Verification items for the finished model (mm, model axes). Give positions to 0.01 mm unless a question says otherwise; leave off trailing zeros. Write each loop counter-clockwise with the first axis right and the second up, starting at its lowest first coordinate (ties: lowest second). Pieces come first, ordered by that corner, then holes.
from build123d import *

# Parameters (mm, degrees)
SKETCH_1_R          = 13
EXTRUDE_1_DEPTH     = 8
SKETCH_6_R          = 14
EXTRUDE_4_DEPTH     = 8
SKETCH_2_R          = 12
CUT_EXTRUDE_1_DEPTH = 3
CUT_EXTRUDE_2_DEPTH = 22.354156504
SKETCH_8_R          = 2.5
CUT_EXTRUDE_3_DEPTH = 2


with BuildPart() as part:
    # 草图1 → 凸台-拉伸1 (new body)
    with BuildSketch(Plane(origin=(0, 0, 0), x_dir=(1, 0, 0), z_dir=(0, 1, 0))):
        with Locations(Location((0, 0, 0), (0, 0, 270))):
            Circle(SKETCH_1_R)
    extrude(amount=EXTRUDE_1_DEPTH)

    # 草图6 → 凸台-拉伸4 (add, through all)
    with BuildSketch(Plane(origin=(0, 8, 0), x_dir=(1, 0, 0), z_dir=(0, 1, 0))):
        with Locations(Location((0, 0, 0), (0, 0, 270))):
            Circle(SKETCH_6_R)
    extrude(amount=-EXTRUDE_4_DEPTH)

    # 草图2 → 切除-拉伸1 (cut)
    with BuildSketch(Plane(origin=(0, 8, 0), x_dir=(1, 0, 0), z_dir=(0, 1, 0))):
        with Locations(Location((0, 0, 0), (0, 0, 270))):
            Circle(SKETCH_2_R)
    extrude(amount=-CUT_EXTRUDE_1_DEPTH, mode=Mode.SUBTRACT)

    # 草图7 → 切除-拉伸2 (cut, through all)
    with BuildSketch(Plane(origin=(0, 8, 0), x_dir=(1, 0, 0), z_dir=(0, 1, 0))):
        Polygon((-15.646830527, 4.142221687), (-12.567085782, 3.326913727), (-12.296421758, 4.349320163), (-15.376166503, 5.164628122), align=None)
        Polygon((-14.689830765, 6.79633564), (-11.798451005, 5.458621977), (-11.354359961, 6.418495447), (-14.245739722, 7.756209109), align=None)
        Polygon((-13.28648793, 9.243946373), (-10.671326264, 7.42447276), (-10.067301683, 8.292647994), (-12.682463348, 10.112121607), align=None)
        Polygon((-11.479441881, 11.410684473), (-9.219958675, 9.164734695), (-8.474353537, 9.914832629), (-10.733836743, 12.160782407), align=None)
        Polygon((-9.3235988, 13.230714699), (-7.488447307, 10.626530804), (-6.623916447, 11.235760092), (-8.45906794, 13.839943987), align=None)
        Polygon((-6.884462888, 14.648736355), (-5.529403257, 11.765445152), (-4.572215008, 12.215294669), (-5.927274639, 15.098585872), align=None)
        Polygon((-4.236146054, 15.621663569), (-3.402351087, 12.546872402), (-2.381589129, 12.8236737), (-3.215384096, 15.898464866), align=None)
        Polygon((-1.459116066, 16.11993444), (-1.171920201, 12.947069284), (-0.11859987, 13.042411894), (-0.405795735, 16.21527705), align=None)
        Polygon((1.362248425, 16.12840926), (1.094118888, 12.953876017), (2.147992986, 12.864863002), (2.416122524, 16.039396246), align=None)
        Polygon((4.142221687, 15.646830527), (3.326913727, 12.567085782), (4.349320163, 12.296421758), (5.164628122, 15.376166503), align=None)
        Polygon((6.79633564, 14.689830765), (5.458621977, 11.798451005), (6.418495447, 11.354359961), (7.756209109, 14.245739722), align=None)
        Polygon((9.243946373, 13.28648793), (7.42447276, 10.671326264), (8.292647994, 10.067301683), (10.112121607, 12.682463348), align=None)
        Polygon((11.410684473, 11.479441881), (9.164734695, 9.219958675), (9.914832629, 8.474353537), (12.160782407, 10.733836743), align=None)
        Polygon((13.230714699, 9.3235988), (10.626530804, 7.488447307), (11.235760092, 6.623916447), (13.839943987, 8.45906794), align=None)
        Polygon((14.648736355, 6.884462888), (11.765445152, 5.529403257), (12.215294669, 4.572215008), (15.098585872, 5.927274639), align=None)
        Polygon((15.621663569, 4.236146054), (12.546872402, 3.402351087), (12.8236737, 2.381589129), (15.898464866, 3.215384096), align=None)
        Polygon((16.11993444, 1.459116066), (12.947069284, 1.171920201), (13.042411894, 0.11859987), (16.21527705, 0.405795735), align=None)
        Polygon((16.12840926, -1.362248425), (12.953876017, -1.094118888), (12.864863002, -2.147992986), (16.039396246, -2.416122524), align=None)
        Polygon((15.646830527, -4.142221687), (12.567085782, -3.326913727), (12.296421758, -4.349320163), (15.376166503, -5.164628122), align=None)
        Polygon((14.689830765, -6.79633564), (11.798451005, -5.458621977), (11.354359961, -6.418495447), (14.245739722, -7.756209109), align=None)
        Polygon((13.28648793, -9.243946373), (10.671326264, -7.42447276), (10.067301683, -8.292647994), (12.682463348, -10.112121607), align=None)
        Polygon((11.479441881, -11.410684473), (9.219958675, -9.164734695), (8.474353537, -9.914832629), (10.733836743, -12.160782407), align=None)
        Polygon((9.3235988, -13.230714699), (7.488447307, -10.626530804), (6.623916447, -11.235760092), (8.45906794, -13.839943987), align=None)
        Polygon((6.884462888, -14.648736355), (5.529403257, -11.765445152), (4.572215008, -12.215294669), (5.927274639, -15.098585872), align=None)
        Polygon((4.236146054, -15.621663569), (3.402351087, -12.546872402), (2.381589129, -12.8236737), (3.215384096, -15.898464866), align=None)
        Polygon((1.459116066, -16.11993444), (1.171920201, -12.947069284), (0.11859987, -13.042411894), (0.405795735, -16.21527705), align=None)
        Polygon((-1.362248425, -16.12840926), (-1.094118888, -12.953876017), (-2.147992986, -12.864863002), (-2.416122524, -16.039396246), align=None)
        Polygon((-4.142221687, -15.646830527), (-3.326913727, -12.567085782), (-4.349320163, -12.296421758), (-5.164628122, -15.376166503), align=None)
        Polygon((-6.79633564, -14.689830765), (-5.458621977, -11.798451005), (-6.418495447, -11.354359961), (-7.756209109, -14.245739722), align=None)
        Polygon((-9.243946373, -13.28648793), (-7.42447276, -10.671326264), (-8.292647994, -10.067301683), (-10.112121607, -12.682463348), align=None)
        Polygon((-11.410684473, -11.479441881), (-9.164734695, -9.219958675), (-9.914832629, -8.474353537), (-12.160782407, -10.733836743), align=None)
        Polygon((-13.230714699, -9.3235988), (-10.626530804, -7.488447307), (-11.235760092, -6.623916447), (-13.839943987, -8.45906794), align=None)
        Polygon((-14.648736355, -6.884462888), (-11.765445152, -5.529403257), (-12.215294669, -4.572215008), (-15.098585872, -5.927274639), align=None)
        Polygon((-15.621663569, -4.236146054), (-12.546872402, -3.402351087), (-12.8236737, -2.381589129), (-15.898464866, -3.215384096), align=None)
        Polygon((-16.11993444, -1.459116066), (-12.947069284, -1.171920201), (-13.042411894, -0.11859987), (-16.21527705, -0.405795735), align=None)
        Polygon((-16.12840926, 1.362248425), (-12.953876017, 1.094118888), (-12.864863002, 2.147992986), (-16.039396246, 2.416122524), align=None)
    extrude(amount=-CUT_EXTRUDE_2_DEPTH, mode=Mode.SUBTRACT)

    # 草图8 → 切除-拉伸3 (cut)
    with BuildSketch(Plane(origin=(0, 5, 0), x_dir=(1, 0, 0), z_dir=(0, 1, 0))):
        with Locations(Location((0, 0, 0), (0, 0, 270))):
            Circle(SKETCH_8_R)
    extrude(amount=-CUT_EXTRUDE_3_DEPTH, mode=Mode.SUBTRACT)


solid = part.part
Item 1: Scan lines: line 1 along X through (y, z) = (4.55, 0); line 2 along X through (y, z) = (5.85, 0); line 3 along Y through (x, z) = (-4.75, -10). Record each from-to range of solid material in increasing order.
Answer key:
line 1: x = -14 to -2.5, 2.5 to 14
line 2: x = -14 to -12, 12 to 14
line 3: y = 0 to 5
Item 2: Release check for a two-part mould opening along Z. For faces 1 (the face through (-10.374, 4.056, -7.852)), 2 (the face through (8.61, 4.06, 11.04)) record: released by +Z, released by -Z, zero draft, split by the parting line, or undercut.
Answer key:
face 1: undercut
face 2: released by +Z
Item 3: Sectioned sample at B-B on x = 1.75. Record the cut outline in (y, z).
Answer key:
outline: (0, -12.9) - (8, -12.9) - (8, -11.87) - (5, -11.87) - (5, -1.79) - (3, -1.79) - (3, 1.79) - (5, 1.79) - (5, 11.87) - (8, 11.87) - (8, 13.89) - (0, 13.89) - close
Item 4: Sectioned sample at A-A on z = 3. Record the cut outline in (x, y), then the cut area to 3 significant figures.
Answer key:
outline: (-12.66, 0) - (13.67, 0) - (13.67, 8) - (11.62, 8) - (11.62, 5) - (-11.62, 5) - (-11.62, 8) - (-12.66, 8) - close
area: 141 mm2
Item 5: Depth check by flat-ended pin: pin 1 (1 mm diameter, centred on x = 8.5, y = 2, fed in from +Z); pin 2 (7 mm diameter, centred on x = -5.5, z = -2, fed in from +Y); pin 3 (1 mm diameter, centred on x = -3.5, y = 4.5, fed in from +Z). Enter the tip coordinate at first touch or a pass-through.
Answer key:
pin 1: stops at z = 11.44
pin 2: stops at y = 5
pin 3: stops at z = 13.67
